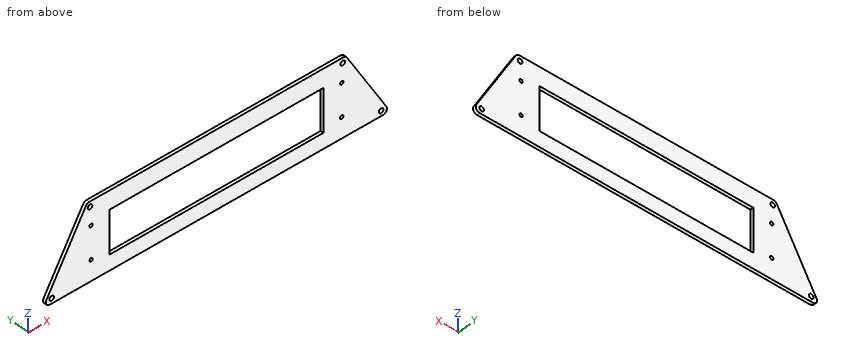
from build123d import *

# Parameters (mm, degrees)
EXTRUDE_1_DEPTH        = 3
HOLE_WIZARD_M4_1_D     = 3.3
HOLE_WIZARD_M4_1_DEPTH = 11.5
HOLE_WIZARD_M4_1_TIP   = 0.991420021
HOLE_WIZARD_M4_2_D     = 4.5
HOLE_WIZARD_M4_2_DEPTH = 8
HOLE_WIZARD_M4_2_TIP   = 1.351936393
FILLET_1_R             = 4
SKETCH_9_W             = 209
SKETCH_9_H             = 42
CUT_EXTRUDE_1_DEPTH    = 172.28583421


with BuildPart() as part:
    # 草图1 → 凸台-拉伸1 (new body)
    with BuildSketch(Plane(origin=(0, 0, 0), x_dir=(1, 0, 0), z_dir=(0, 1, 0))):
        Polygon((-169.688021535, 36), (-126.386751346, -39), (126.386751346, -39), (169.688021535, 36), align=None)
    extrude(amount=EXTRUDE_1_DEPTH)

    # M4 螺纹孔1
    with Locations(Plane(origin=(0, 3, 0), x_dir=(1, 0, 0), z_dir=(0, 1, 0))):
        with Locations((122.5, 16), (-122.5, -16), (-122.5, 16), (122.5, -16)):
            Hole(HOLE_WIZARD_M4_1_D / 2, depth=HOLE_WIZARD_M4_1_DEPTH)
            with Locations((0, 0, -(HOLE_WIZARD_M4_1_DEPTH + HOLE_WIZARD_M4_1_TIP / 2))):  # 118° drill point
                Cone(0, HOLE_WIZARD_M4_1_D / 2, HOLE_WIZARD_M4_1_TIP, mode=Mode.SUBTRACT)

    # M4 间隙孔2
    with Locations(Plane(origin=(0, 0, 0), x_dir=(-1, 0, 0), z_dir=(0, -1, 0))):
        with Locations((-123.5, -34), (123.5, -34), (161.027767497, 31), (-161.027767497, 31)):
            Hole(HOLE_WIZARD_M4_2_D / 2, depth=HOLE_WIZARD_M4_2_DEPTH)
            with Locations((0, 0, -(HOLE_WIZARD_M4_2_DEPTH + HOLE_WIZARD_M4_2_TIP / 2))):  # 118° drill point
                Cone(0, HOLE_WIZARD_M4_2_D / 2, HOLE_WIZARD_M4_2_TIP, mode=Mode.SUBTRACT)

    # 圆角1
    fillet_1_edges = [part.edges().sort_by_distance(p)[0] for p in [
        (169.688021535, 1.5, -36),
        (126.386751346, 1.5, 39),
        (-126.386751346, 1.5, 39),
        (-169.688021535, 1.5, -36),
    ]]
    fillet(fillet_1_edges, radius=FILLET_1_R)

    # 草图9 → 切除-拉伸1 (cut, through all)
    with BuildSketch(Plane.XZ):
        Rectangle(SKETCH_9_W, SKETCH_9_H)
    extrude(amount=-CUT_EXTRUDE_1_DEPTH, mode=Mode.SUBTRACT)


solid = part.part
Geometry: final body of the model. Coordinates: model frame, mm. Give positions to 0.01 mm unless a question says otherwise; leave off trailing zeros. Write each loop counter-clockwise with the first axis right and the second up, starting at its lowest first coordinate (ties: lowest second). Pieces come first, ordered by that corner, then holes.
(1) Ray query, line 1 (Z direction, x = 42.5, y = 2.8); line 2 (X direction, y = 0.75, z = -32); line 3 (X direction, y = 0.4, z = 33). Return the intervals inside material, ascending.
(2) Cut plane B-B, the plane z = -5. Return loops of the section in (x, y).
(3) Cut plane D-D, the plane z = 25. Return loops of the section in (x, y), then the cut area to 3 significant figures.
(4) Cut plane C-C, the plane y = 1.65. Give the number of separate pieces and of enclosed holes in the cut face, then the cut area to 3 significant figures.
(5) First-contact query: P1, Ø4, axis at x = -161.03, z = -31, coming from the -Y side; P2, Ø1.5, axis at y = 1, z = -9, coming from the +X side; P3, Ø1.5, axis at y = 2, z = 9.5, coming from the -X side; P4, Ø7, axis at x = -123.5, z = 34, coming from the +Y side. Flat tips, straight axial feed; report the tip coordinate or a pass-through.
(6) Cut plane A-A, the plane x = -44. Return loops of the section in (y, z).
Values follow:
1. line 1: z = -36 to -21, 21 to 39
1. line 2: x = -166.76 to -163.04, -159.01 to 159.01, 163.04 to 166.76
1. line 3: x = -129.85 to -125.52, -121.48 to 121.48, 125.52 to 129.85
2. outline: (-151.79, 0) - (-104.5, 0) - (-104.5, 3) - (-151.79, 3) - close; (104.5, 0) - (151.79, 0) - (151.79, 3) - (104.5, 3) - close
3. outline: (-134.47, 0) - (134.47, 0) - (134.47, 3) - (-134.47, 3) - close
3. area: 807 mm2
4. separate pieces: 1
4. enclosed holes: 9
4. area: 13,300 mm2
5. P1: passes through
5. P2: stops at x = 154.53
5. P3: stops at x = -143.85
5. P4: stops at y = 3
6. outline: (0, -36) - (3, -36) - (3, -21) - (0, -21) - close; (0, 21) - (3, 21) - (3, 39) - (0, 39) - close
